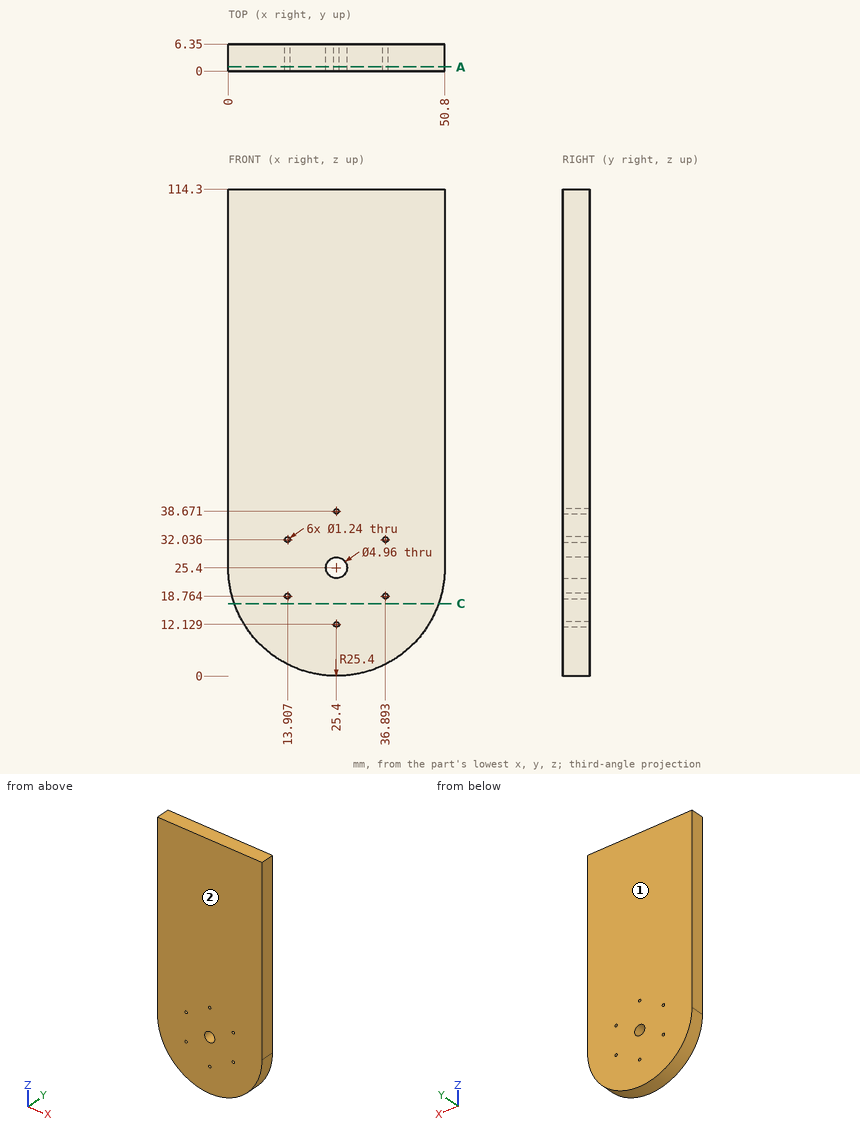
Can you work these out from the drawing? Everything is in mm from the part's minimum corner. Round coordinates to 2 decimals unless told otherwise and drop trailing zeros. Write each loop counter-clockwise with the first axis right and the second up, starting at its lowest first coordinate (ties: lowest second). Pieces come first, ordered by that corner, then holes.
1. Will these pins go through, and if not, where does the flat tip stop? pin 1 Ø2 at (x, z) = (13.91, 32.04) entering from -Y; pin 2 Ø1.1 at (x, z) = (36.89, 18.76) entering from -Y; pin 3 Ø2 at (y, z) = (5.5, 14.5) entering from -X.
2. If we mould it in two halves opening along Y, with no side actions, what happens to the marked faces 1 and 2? For each: released by +Y, released by -Y, zero draft, split by the parting line, or undercut.
3. I need wall thicknesses on L1, parallel to Z at x = 36.5, y = 1.5 (1 decimal); L2, parallel to Z at x = 14, y = 4; L3, parallel to Z at x = 24.5, y = 2.75 (1 decimal). Which ranges of each line are inside material? Lowest first, please.
4. Suppose I cut it at A-A (y = 1). State how many separate pieces and enclosed holes the cut face has, and give its area (3 significant figures).
5. Suppose I cut it at C-C (z = 17). List the corners of the cut face in (x, y) for me.
Answer sheet:
1. pin 1: stops at y = 0
1. pin 2: passes through
1. pin 3: stops at x = 2.01
2. face 1: released by +Y
2. face 2: released by -Y
3. L1: z = 2.6 to 18.3, 19.2 to 31.6, 32.5 to 114.3
3. L2: z = 2.7 to 18.15, 19.38 to 31.42, 32.65 to 114.3
3. L3: z = 0 to 23.1, 27.7 to 114.3
4. separate pieces: 1
4. enclosed holes: 7
4. area: 5,500 mm2
5. outline: (1.43, 0) - (49.37, 0) - (49.37, 6.35) - (1.43, 6.35) - close
